```python
from build123d import *

# Parameters (mm, degrees)
F1_DEPTH = 76.2
F2_DEPTH = 76.2
F3_W     = 139.7
F3_H     = 76.2
F4_DEPTH = 6.35


with BuildPart() as f1:
    # F0 (on Right) → F1 (new body)
    with BuildSketch(Plane.YZ):
        with BuildLine():
            Line((-44.45, 0), (44.45, 0))
            add(Edge.make_bspline(
                [(0, 63.5), (22.225, 63.5), (44.45, 43.3620624244), (44.45, 0)],
                knots=[0.5, 0.5, 0.5, 0.5, 1, 1, 1, 1], degree=3))
            add(Edge.make_bspline(
                [(-44.45, 0), (-44.45, 43.3620624244), (-22.225, 63.5), (0, 63.5)],
                knots=[0, 0, 0, 0, 0.5, 0.5, 0.5, 0.5], degree=3))
        make_face()
    extrude(amount=F1_DEPTH)

    # F2 (add): a face of the model
    f2_faces = [f1.faces().sort_by_distance(p)[0] for p in [
        (0, 0, 27.2904966015),
    ]]
    extrude(f2_faces, amount=F2_DEPTH)

    # F3 (on face) → F4 (cut)
    with BuildSketch(Plane(origin=(0, 0, 0), x_dir=(1, 0, 0), z_dir=(0, 0, -1))):
        Polygon((76.2, -44.45), (76.2, 44.45), (0, 44.45), (-76.2, 44.45), (-76.2, -44.45), (0, -44.45), align=None)
        Rectangle(F3_W, F3_H, mode=Mode.SUBTRACT)
    extrude(amount=-F4_DEPTH, mode=Mode.SUBTRACT)


solid = f1.part
```
Verification items for the finished model (mm, model axes). A direction names the side the tool comes from. Coordinates: 2 decimals unless noted, no trailing zeros. Write item = value, one per line.
Q1. Material ranges on L1, parallel to Y at x = 36, z = 5; L2, parallel to X at y = -25, z = 5; L3, parallel to Z at x = 1, y = -18, recorded low to high. Write a range as from..to.
Answer:
L1 = -38.1..38.1
L2 = -69.85..69.85
L3 = 0..58.8
Q2. Access from +Z, -Z, +X, -X, +Y, -Y to the whole of each face (thin tool, end or side, straight path). Record for faces 1 (the face through (69.85, 1, 3)), 2 (the face through (-1, -38.1, 3)), 3 (the face through (-69.85, 1, 3)), 4 (the face through (-1, 38.1, 3)).
Answer:
face_1 = -Z, +X, +Y, -Y
face_2 = -Z, +X, -X, -Y
face_3 = -Z, -X, +Y, -Y
face_4 = -Z, +X, -X, +Y
Q3. Go/stop test with flat-tipped pins: pin 1 Ø7 at (y, z) = (13, 3) entering from -X; pin 2 Ø5 at (x, z) = (30.5, 2.5) entering from +Y; pin 3 Ø6 at (x, y) = (43.5, -20) entering from +Z; pin 4 Ø3 at (y, z) = (16, 3) entering from +X. Record where each tip stops, or that it passes through.
Answer:
pin_1 = -76.2
pin_2 = 38.1
pin_3 = 59.33
pin_4 = 69.85
